Geometry check sheet. Reference: the model listing, model coordinates, mm. Face numbers are marked on the shaded views. A direction names the side the tool comes from. Coordinates: 2 decimals unless noted, no trailing zeros. Loops run counter-clockwise (first coordinate to the right, second up) from the corner with the lowest first, then second, coordinate; pieces in that order, holes last. Notation, with made-up numbers: (68, 58) - (75, 58) arc R15 ccw to (75, 72) - close; hole circle Ø4 at (65.5, 51.25). An arc over 180 degrees is marked (long way). One line per item, written item: value.
Autodesk Inventor part; units mm, degrees
ref_plane "YZ Plane" through (0, 0, 0) normal (1, 0, 0) x (0, 1, 0)
ref_plane "XZ Plane" through (0, 0, 0) normal (0, 1, 0) x (-1, 0, 0)
ref_plane "XY Plane" through (0, 0, 0) normal (0, 0, 1) x (1, 0, 0)
sketch "Sketch1" plane through (0, 0, 0) normal (0, 1, 0) x (-1, 0, 0)
  circle A0 centre (25, 36.3) radius 2.5
  circle A1 centre (33, 49.9) radius 2.5
  line L0 (15, 0) -> (15, 15)
  line L1 (15, 15) -> (0, 15)
  line L2 (0, 15) -> (0, 80)
  line L3 (0, 80) -> (41, 80)
  line L4 (41, 80) -> (41, 0)
  line L5 (15, 0) -> (41, 0)
  circle A2 centre (25, 36.3) radius 7.5 construction
  circle A3 centre (33, 49.9) radius 7.5 construction
  point P0 (0, 0)
  dimension "d0" = 5
  dimension "d1" = 15
  dimension "d2" = 25
  dimension "d3" = 21.3
  dimension "d4" = 8
  dimension "d5" = 13.6
  dimension "d12" = 15
  dimension "d46" = 80
  dimension "d47" = 41
extrude "Extrusion1" add sketch "Sketch1" along normal blind 3
sketch "Sketch2" plane through (0, 3, 0) normal (0, 1, 0) x (1, 0, 0)
  line L0 (-41, 0) -> (-41, -80)
  line L1 (-41, -80) -> (0, -80)
  line L2 (0, -80) -> (0, -15)
  line L3 (0, -15) -> (-15, -15)
  line L4 (-15, -15) -> (-15, 0)
  line L5 (-15, 0) -> (-41, 0)
  circle A0 centre (-33, -49.9) radius 2.5
  circle A1 centre (-25, -36.3) radius 2.5
  line L6 (-15, -15) -> (-15, 0)
  line L7 (-15, -15) -> (-15, -80)
  line L8 (-15, -15) -> (-41, -15)
  line L9 (-41, 0) -> (-41, -80)
  point P0 (0, 0)
extrude "Extrusion2" add sketch "Sketch2" along normal blind 3 contours L5 L4 L8 L0 | L3 L2 L1 L7
sketch "Sketch3" plane through (0, 3, 0) normal (0, 1, 0) x (1, 0, 0)
  circle A0 centre (-25, -36.3) radius 2.5
  circle A1 centre (-33, -49.9) radius 2.5
  line L0 (-15, -80) -> (-15, -15)
  line L1 (-15, -15) -> (-41, -15)
  line L2 (-41, -15) -> (-41, -80)
  line L3 (-41, -80) -> (-15, -80)
  circle A2 centre (-25, -36.3) radius 2.5
  circle A3 centre (-25, -36.3) radius 8.5
  circle A4 centre (-33, -49.9) radius 2.5
  circle A5 centre (-33, -49.9) radius 8.5
  line L4 (-31.8739, -31.3) -> (-41, -31.3)
  line L5 (-41, 0) -> (-41, -80)
  line L6 (-33, -41.4) -> (-41, -41.4)
  line L7 (-38.3753, -56.4846) -> (-41, -56.4846)
  line L8 (-29, -57.4) -> (-29, -80)
  line L9 (-41, -80) -> (0, -80)
  point P0 (0, 0)
  point P1 (-31.727, -41.4959)
  dimension "d15" = 17
  dimension "d16" = 5
  dimension "d19" = 12
extrude "Extrusion3" add sketch "Sketch3" along normal blind 21 contours L3 L2 L7 A5 L8 | L4 A3 A5 L6 L2
fillet "Fillet1" radius 1 8 edges at (-31.8739, 13.5, 31.3) (-31.727, 13.5, 41.4959) (-41, 13.5, 41.4) (-41, 13.5, 31.3) (-41, 13.5, 56.4846) (-29, 13.5, 57.4) (-29, 13.5, 80) (-38.3753, 13.5, 56.4846)
chamfer "Chamfer1" distance 10 angle 45 1 edges at (-41, 12, 80)
sketch "Sketch4" plane through (0, 24, 0) normal (0, 1, 0) x (1, 0, 0)
  line L0 (-31, -80) -> (-41, -70)
  line L1 (-31, -80) -> (-30, -80)
  arc A0 (-30, -80) -> (-29, -79) centre (-30, -79) ccw
  line L2 (-29, -79) -> (-29, -58.9139)
  arc A1 (-29, -58.9139) -> (-30.3158, -57.965) centre (-30, -58.9139) ccw
  arc A2 (-38.1184, -56.6862) -> (-30.3158, -57.965) centre (-33, -49.9) ccw
  arc A3 (-38.1184, -56.6862) -> (-38.7205, -56.4846) centre (-38.7205, -57.4846) ccw
  line L3 (-38.7205, -56.4846) -> (-40, -56.4846)
  arc A4 (-40, -56.4846) -> (-41, -57.4846) centre (-40, -57.4846) ccw
  line L4 (-41, -57.4846) -> (-41, -70)
  arc A5 (-40, -31.3) -> (-41, -32.3) centre (-40, -32.3) ccw
  line L5 (-41, -32.3) -> (-41, -40.4)
  arc A6 (-41, -40.4) -> (-40, -41.4) centre (-40, -40.4) ccw
  line L6 (-40, -41.4) -> (-33.5697, -41.4)
  arc A7 (-33.5697, -41.4) -> (-32.6676, -39.9684) centre (-33.5697, -40.4) ccw
  arc A8 (-32.7098, -32.7211) -> (-32.6676, -39.9684) centre (-25, -36.3) ccw
  arc A9 (-32.7098, -32.7211) -> (-33.6168, -31.3) centre (-33.6168, -32.3) ccw
  line L7 (-33.6168, -31.3) -> (-40, -31.3)
  point P0 (0, 0)
  point P1 (-37, -36)
  point P2 (-37, -66)
  dimension "d24" = 4
  dimension "d25" = 36
  dimension "d26" = 30
hole "Hole1" at (-37, 24, 36) at (-37, 24, 66) direction (0, -1, 0) diameter 2.8 depth 10 tip angle 118
sketch "Sketch5" plane through (0, 0, 0) normal (0, -1, 0) x (1, 0, 0)
  line L0 (-41, 70) -> (-31, 80)
  line L1 (-41, 0) -> (-41, 70)
  line L2 (-15, 0) -> (-41, 0)
  line L3 (-15, 15) -> (-15, 0)
  line L4 (0, 15) -> (-15, 15)
  line L5 (0, 80) -> (0, 15)
  line L6 (-31, 80) -> (0, 80)
  circle A0 centre (-33, 49.9) radius 2.5
  circle A1 centre (-25, 36.3) radius 2.5
  point P0 (0, 0)
  point P1 (-31, 7.5)
  point P2 (-7.5, 25)
  point P3 (-7.5, 65)
  dimension "d34" = 7.5
  dimension "d35" = 7.5
  dimension "d36" = 10
  dimension "d37" = 15
  dimension "d38" = 40
hole "Hole2" at (-31, 0, 7.5) at (-7.5, 0, 25) at (-7.5, 0, 65) direction (0, 1, 0) diameter 3.6 end through all counterbore diameter 6.5 counterbore depth 3.4
properties part number "Alpha Idler Assembly" material "ABS Plastic"
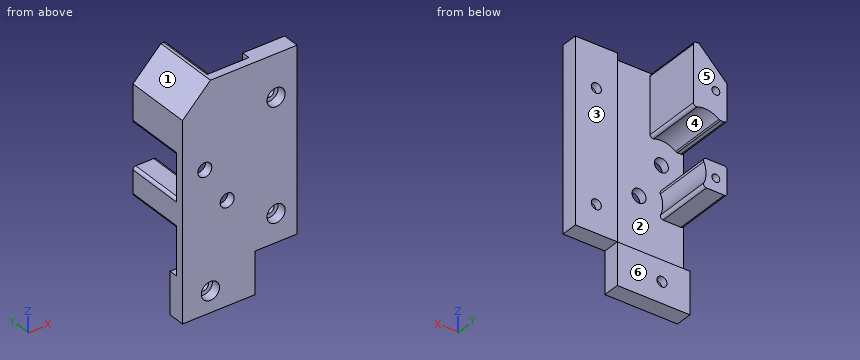
(1) Cross-section at C-C on y = 16.25. State how many separate pieces and enclosed holes the cut face has, and give its area (3 significant figures).
Reply:
separate pieces: 2
enclosed holes: 2
area: 285 mm2
(2) Go/stop test with flat-tipped pins: pin 1 Ø4 at (x, z) = (-7.5, 25) entering from -Y; pin 2 Ø6 at (x, z) = (-31, 7.5) entering from +Y; pin 3 Ø2 at (x, y) = (-8, 5.5) entering from -Z. Record where each tip stops, or that it passes through.
Reply:
pin 1: y = 3.4
pin 2: y = 6
pin 3: z = 15
(3) Access from +Z, -Z, +X, -X, +Y, -Y to the whole of each face (thin tool, end or side, straight path). Record for the marked faces 4, 5 and 6.
Reply:
face 4: +Y
face 5: +Z, -Z, +X, -X, +Y
face 6: -Z, +X, -X, +Y
(4) Cross-section at D-D on z = 25. Record the cut outline in (x, y).
Reply:
outline: (-41, 0) - (-10.75, 0) - (-10.75, 3.4) - (-9.3, 3.4) - (-9.3, 6) - (-15, 6) - (-15, 3) - (-41, 3) - close; (-5.7, 3.4) - (-4.25, 3.4) - (-4.25, 0) - (0, 0) - (0, 6) - (-5.7, 6) - close
(5) Release check for a two-part mould opening along X. For the marked faces 1, 2 and 3 record: pulls with the +X half, pulls with the -X half, needs draft (parallel to the pull), parting line crosses it, or undercut.
Reply:
face 1: pulls with the -X half
face 2: undercut
face 3: needs draft
(6) Material ranges on probe 1 along X at (y, z) = (20.75, 66); probe 2 along X at (y, z) = (5.35, 7.5); probe 3 along Z at (x, y) = (-37.5, 20.5), recorded low to high. Write a range as from..to.
Reply:
probe 1: -41..-38.4, -35.6..-29
probe 2: -41..-32.8, -29.2..-15
probe 3: 31.3..34.69, 37.31..41.4, 57.11..64.69, 67.31..73.5
(7) Cross-section at B-B on x = -25. Record the cut outline in (y, z).
Reply:
outline: (0, 0) - (6, 0) - (6, 15) - (3, 15) - (3, 33.8) - (0, 33.8) - close; (0, 38.8) - (3, 38.8) - (3, 80) - (0, 80) - close
(8) Cross-section at A-A on z = 7.5. Record the cut outline in (x, y).
Reply:
outline: (-41, 0) - (-34.25, 0) - (-34.25, 3.4) - (-32.8, 3.4) - (-32.8, 6) - (-41, 6) - close; (-29.2, 3.4) - (-27.75, 3.4) - (-27.75, 0) - (-15, 0) - (-15, 6) - (-29.2, 6) - close
